```python
from build123d import *

# Parameters (mm, degrees)
F1_DEPTH = 25
F2_W     = 10.574922
F2_H     = 25.480952
F3_DEPTH = 23.4
F4_R     = 10.767278
F4_R_2   = 5.787824
F5_DEPTH = 25


with BuildPart() as f1:
    # F0 (on Front) → F1 (new body)
    with BuildSketch(Plane.XZ):
        Polygon((-76.671138, -50.506882), (-101.848751, -50.506882), (-102.75878, -70.527636), (-54.223638, -70.527636), (-54.223638, 48.080128), (22.522558, 48.080128), (22.522558, -71.134321), (73.181108, -71.134321), (73.181108, -45.653369), (37.083104, -40.193167), (37.083104, 62.033977), (-76.671138, 62.033977), align=None)
    extrude(amount=F1_DEPTH)

    # F2 (on face) → F3 (cut)
    with BuildSketch(Plane.YZ.offset(73.181108)):
        with Locations((-13.039805, -58.393845)):
            Rectangle(F2_W, F2_H)
    extrude(amount=-F3_DEPTH, mode=Mode.SUBTRACT)

    # F4 (on face) → F5 (join)
    with BuildSketch(Plane.YZ.offset(37.083104)):
        with Locations((-13.808914, 11.681821)):
            Circle(F4_R)
        with Locations((-13.808914, 11.681821)):
            Circle(F4_R_2, mode=Mode.SUBTRACT)
    extrude(amount=F5_DEPTH)


solid = f1.part
```
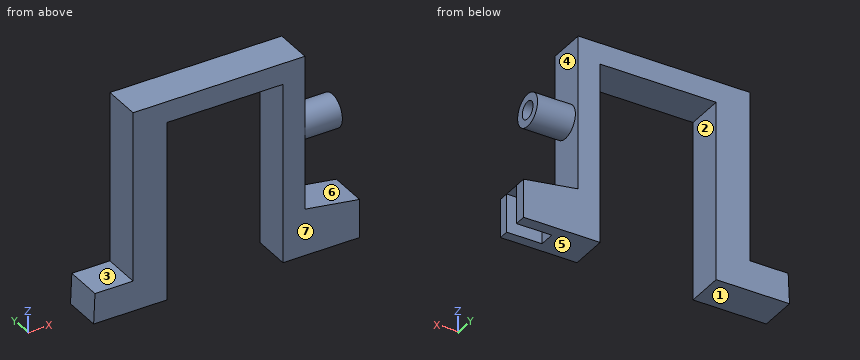
The model under review builds one solid part; all positions refer to its coordinate system, in mm. Face numbers are marked on the shaded views. A direction names the side the tool comes from. Round coordinates to 2 decimals unless told otherwise and drop trailing zeros. Order: outer loops, then holes, each group sorted by start corner. A loop starts at its lowest first (then second) coordinate and runs counter-clockwise, first axis right, second up. Notation, with made-up numbers: (52, -4) -> (66, -4) arc R17 cw to (66, 19) -> close; hole circle Ø11 at (0, 20.5). An arc over 180 degrees is marked (long way). Use a Markdown table: item, result.
Q1. We need section B-B on x = 52. Write out the cut boundary in (y, z), then the cut area to 3 significant figures.
Values:
| item | result |
|---|---|
| outline | (-25, -71.13) -> (-18.33, -71.13) -> (-18.33, -45.65) -> (-7.75, -45.65) -> (-7.75, -71.13) -> (0, -71.13) -> (0, -42.45) -> (-25, -42.45) -> close; circle Ø21.53 at (-13.81, 11.68); hole circle Ø11.58 at (-13.81, 11.68) |
| area | 707 mm^2 |
Q2. Mouldability with a two-part tool opening along Z and no side actions: class the marked faces 4, 5, 6 and 7 as +Z half, -Z half, draft (parallel to the pull), parting line (faces both ways), or undercut.
Values:
| item | result |
|---|---|
| face 4 | undercut |
| face 5 | -Z half |
| face 6 | undercut |
| face 7 | draft |
Q3. Clearance check with flat-ended pins moving along their axes: P1, Ø5.5, axis at x = 57, y = -13, coming from the -Z side; P2, Ø3, axis at y = -14.5, z = -61.5, coming from the +X side; P3, Ø4, axis at x = -6, y = -9.5, coming from the -Z side; P4, Ø7, axis at x = 56.5, z = -58, coming from the +Y side. State where each tip first meets the part, or that it passes through.
Values:
| item | result |
|---|---|
| P1 | stops at z = -45.65 |
| P2 | stops at x = 49.78 |
| P3 | stops at z = 48.08 |
| P4 | stops at y = 0 |
Q4. We need section A-A on z = -21. Write out the cut boundary in (x, y), then the cut area to 3 significant figures.
Values:
| item | result |
|---|---|
| outline | (-76.67, -25) -> (-54.22, -25) -> (-54.22, 0) -> (-76.67, 0) -> close; (22.52, -25) -> (37.08, -25) -> (37.08, 0) -> (22.52, 0) -> close |
| area | 925 mm^2 |
Q5. We need section D-D on y = -11.75. Write out the cut boundary in (x, z).
Values:
| item | result |
|---|---|
| outline | (-102.76, -70.53) -> (-54.22, -70.53) -> (-54.22, 48.08) -> (22.52, 48.08) -> (22.52, -71.13) -> (49.78, -71.13) -> (49.78, -45.65) -> (73.18, -45.65) -> (37.08, -40.19) -> (37.08, 1.11) -> (62.08, 1.11) -> (62.08, 6.27) -> (37.08, 6.27) -> (37.08, 17.09) -> (62.08, 17.09) -> (62.08, 22.25) -> (37.08, 22.25) -> (37.08, 62.03) -> (-76.67, 62.03) -> (-76.67, -50.51) -> (-101.85, -50.51) -> close |
Q6. We need section C-C on z = 13.5. Write out the cut boundary in (x, y).
Values:
| item | result |
|---|---|
| outline | (-76.67, -25) -> (-54.22, -25) -> (-54.22, 0) -> (-76.67, 0) -> close; (22.52, -25) -> (37.08, -25) -> (37.08, -24.42) -> (62.08, -24.42) -> (62.08, -19.3) -> (37.08, -19.3) -> (37.08, -8.31) -> (62.08, -8.31) -> (62.08, -3.2) -> (37.08, -3.2) -> (37.08, 0) -> (22.52, 0) -> close |
Q7. Tool access review of the marked faces 1, 2 and 3: name each direction out of +Z, -Z, +X, -X, +Y, -Y from which nothing blocks a thin tool from reaching the whole face with its end or side.
Values:
| item | result |
|---|---|
| face 1 | -Z, -X, +Y, -Y |
| face 2 | -Z, +Y, -Y |
| face 3 | +Z, -X, +Y, -Y |
Q8. For line 1 (X direction, y = -3, z = 46); line 2 (X direction, y = -15.5, z = 18); line 3 (Y direction, x = 57.5, z = -50), list the stretches that pass through material, from the lowest coordinate up.
Values:
| item | result |
|---|---|
| line 1 | x = -76.67 to -54.22, 22.52 to 37.08 |
| line 2 | x = -76.67 to -54.22, 22.52 to 62.08 |
| line 3 | y = -25 to -18.33, -7.75 to 0 |
